Verification items for the finished model (mm, model axes). Coordinates: 2 decimals unless noted, no trailing zeros. Return JSON: item names as keys, results as strings. Group by question number.
Q1. Section check A-A, the plane y = 2. Count the separate pieces of the cut face and the enclosed holes in it, then the cut area to 3 significant figures.
Q2. Thickness scan on probe 1 along Z at (x, y) = (-91.5, 1.9) (3 decimals); probe 2 along X at (y, z) = (3.1, -29.5); probe 3 along Z at (x, y) = (-35.5, 0.8) (3 decimals). Record the ranges inside material, lowest first.
Q3. Mould release check, pull along Z, two halves, no side actions. Record for faces 1 (the face through (38.98, 2.46, 2.05)), 2 (the face through (153.225, 2.535, 1.55)): pulls with the +Z half, pulls with the -Z half, needs draft (parallel to the pull), parting line crosses it, or undercut.
Q4. Go/stop test with flat-tipped pins: pin 1 Ø1.5 at (y, z) = (3, -15.5) entering from -X; pin 2 Ø6 at (x, z) = (45.5, -21) entering from +Y; pin 3 Ø1.8 at (x, z) = (-105, -20.125) entering from +Y; pin 4 Ø2.5 at (x, y) = (-62.5, 3) entering from +Z (3 decimals). Record where each tip stops, or that it passes through.
from build123d import *

# Parameters (mm, degrees)
EXTRUDE_1_DEPTH      = 5
SKETCH_2_R           = 1.525
CUT_EXTRUDE_1_DEPTH  = 6
SKETCH_3_R           = 48.25
EXTRUDE_2_DEPTH      = 5
SKETCH_6_R           = 1.525
CUT_EXTRUDE_4_DEPTH  = 6
SKETCH_7_R           = 1.775
CUT_EXTRUDE_5_DEPTH  = 6
FILLET_1_R           = 40
SKETCH_9_R           = 14
CUT_EXTRUDE_7_DEPTH  = 6
SKETCH_10_R          = 8
CUT_EXTRUDE_8_DEPTH  = 6
SKETCH_11_R          = 15
CUT_EXTRUDE_9_DEPTH  = 6
SKETCH_12_R          = 3
CUT_EXTRUDE_10_DEPTH = 6
SKETCH_13_R          = 1.525
CUT_EXTRUDE_11_DEPTH = 6
SKETCH_18_R          = 1.525
CUT_EXTRUDE_13_DEPTH = 6
SKETCH_21_R          = 1.525
CUT_EXTRUDE_15_DEPTH = 6
CUT_EXTRUDE_16_DEPTH = 6


with BuildPart() as part:
    # 草图1 → 凸台-拉伸1 (new body)
    with BuildSketch(Plane(origin=(0, 0, 0), x_dir=(1, 0, 0), z_dir=(0, 1, 0))):
        with BuildLine():
            ThreePointArc((-78.875, 0), (-86.526835342, -18.473164658), (-105, -26.125))
            Line((-105, -26.125), (105, -26.125))
            Line((105, -26.125), (105, 26.125))
            Line((105, 26.125), (-105, 26.125))
            ThreePointArc((-105, 26.125), (-86.526835342, 18.473164658), (-78.875, 0))
        make_face()
        with BuildLine():
            ThreePointArc((-105, 26.125), (-131.125, 0), (-105, -26.125))
            Line((-105, -26.125), (-105, 26.125))
        make_face()
        with BuildLine():
            Line((-105, 26.125), (-105, -26.125))
            ThreePointArc((-105, -26.125), (-86.526835342, -18.473164658), (-78.875, 0))
            ThreePointArc((-78.875, 0), (-86.526835342, 18.473164658), (-105, 26.125))
        make_face()
    extrude(amount=EXTRUDE_1_DEPTH)

    # 草图2 → 切除-拉伸1 (cut, through all)
    with BuildSketch(Plane(origin=(0, 5, 0), x_dir=(1, 0, 0), z_dir=(0, 1, 0))):
        with Locations((-91.5, 0)):
            Circle(SKETCH_2_R)
        with Locations((-98.25, -11.691342951)):
            Circle(SKETCH_2_R)
        with Locations((-111.75, -11.691342951)):
            Circle(SKETCH_2_R)
        with Locations((-118.5, 0)):
            Circle(SKETCH_2_R)
        with Locations((-111.75, 11.691342951)):
            Circle(SKETCH_2_R)
        with Locations((-98.25, 11.691342951)):
            Circle(SKETCH_2_R)
    extrude(amount=-CUT_EXTRUDE_1_DEPTH, mode=Mode.SUBTRACT)

    # 草图3 → 凸台-拉伸2 (add)
    with BuildSketch(Plane(origin=(0, 5, 0), x_dir=(1, 0, 0), z_dir=(0, 1, 0))):
        with Locations((105, 0)):
            Circle(SKETCH_3_R)
    extrude(amount=-EXTRUDE_2_DEPTH)

    # 草图6 → 切除-拉伸4 (cut, through all)
    with BuildSketch(Plane(origin=(0, 5, 0), x_dir=(1, 0, 0), z_dir=(0, 1, 0))):
        with Locations((118.435028843, 13.435028843)):
            Circle(SKETCH_6_R)
        with Locations((124, 0)):
            Circle(SKETCH_6_R)
        with Locations((118.435028843, -13.435028843)):
            Circle(SKETCH_6_R)
        with Locations((105, -19)):
            Circle(SKETCH_6_R)
        with Locations((91.564971157, -13.435028843)):
            Circle(SKETCH_6_R)
        with Locations((86, 0)):
            Circle(SKETCH_6_R)
        with Locations((91.564971157, 13.435028843)):
            Circle(SKETCH_6_R)
        with Locations((105, 19)):
            Circle(SKETCH_6_R)
    extrude(amount=-CUT_EXTRUDE_4_DEPTH, mode=Mode.SUBTRACT)

    # 草图7 → 切除-拉伸5 (cut, through all)
    with BuildSketch(Plane(origin=(0, 5, 0), x_dir=(1, 0, 0), z_dir=(0, 1, 0))):
        with Locations((149.5, 0)):
            Circle(SKETCH_7_R)
        with Locations((136.466251763, -31.466251763)):
            Circle(SKETCH_7_R)
        with Locations((105, -44.5)):
            Circle(SKETCH_7_R)
        with Locations((73.533748237, -31.466251763)):
            Circle(SKETCH_7_R)
        with Locations((60.5, 0)):
            Circle(SKETCH_7_R)
        with Locations((73.533748237, 31.466251763)):
            Circle(SKETCH_7_R)
        with Locations((105, 44.5)):
            Circle(SKETCH_7_R)
        with Locations((136.466251763, 31.466251763)):
            Circle(SKETCH_7_R)
    extrude(amount=-CUT_EXTRUDE_5_DEPTH, mode=Mode.SUBTRACT)

    # 圆角1
    fillet_1_edges = [part.edges().sort_by_distance(p)[0] for p in [
        (64.43465919, 2.5, 26.125),
        (64.43465919, 2.5, -26.125),
    ]]
    fillet(fillet_1_edges, radius=FILLET_1_R)

    # 草图9 → 切除-拉伸7 (cut, through all)
    with BuildSketch(Plane(origin=(0, 5, 0), x_dir=(1, 0, 0), z_dir=(0, 1, 0))):
        with Locations((105, 0)):
            Circle(SKETCH_9_R)
    extrude(amount=-CUT_EXTRUDE_7_DEPTH, mode=Mode.SUBTRACT)

    # 草图10 → 切除-拉伸8 (cut, through all)
    with BuildSketch(Plane(origin=(0, 5, 0), x_dir=(1, 0, 0), z_dir=(0, 1, 0))):
        with Locations((-105, 0)):
            Circle(SKETCH_10_R)
    extrude(amount=-CUT_EXTRUDE_8_DEPTH, mode=Mode.SUBTRACT)

    # 草图11 → 切除-拉伸9 (cut, through all)
    with BuildSketch(Plane(origin=(0, 5, 0), x_dir=(1, 0, 0), z_dir=(0, 1, 0))):
        with Locations((105, 0)):
            Circle(SKETCH_11_R)
    extrude(amount=-CUT_EXTRUDE_9_DEPTH, mode=Mode.SUBTRACT)

    # 草图12 → 切除-拉伸10 (cut, through all)
    with BuildSketch(Plane(origin=(0, 5, 0), x_dir=(1, 0, 0), z_dir=(0, 1, 0))):
        with Locations((117.437211552, 30.026084807)):
            Circle(SKETCH_12_R)
        with Locations((135.026084807, 12.437211552)):
            Circle(SKETCH_12_R)
        with Locations((135.026084807, -12.437211552)):
            Circle(SKETCH_12_R)
        with Locations((117.437211552, -30.026084807)):
            Circle(SKETCH_12_R)
        with Locations((92.562788448, -30.026084807)):
            Circle(SKETCH_12_R)
        with Locations((74.973915193, -12.437211552)):
            Circle(SKETCH_12_R)
        with Locations((74.973915193, 12.437211552)):
            Circle(SKETCH_12_R)
        with Locations((92.562788448, 30.026084807)):
            Circle(SKETCH_12_R)
    extrude(amount=-CUT_EXTRUDE_10_DEPTH, mode=Mode.SUBTRACT)

    # 草图13 → 切除-拉伸11 (cut, through all)
    with BuildSketch(Plane(origin=(0, 5, 0), x_dir=(1, 0, 0), z_dir=(0, 1, 0))):
        with Locations((122.02941274, 41.112639197)):
            Circle(SKETCH_13_R)
        with Locations((146.112639197, 17.02941274)):
            Circle(SKETCH_13_R)
        with Locations((146.112639197, -17.02941274)):
            Circle(SKETCH_13_R)
        with Locations((122.02941274, -41.112639197)):
            Circle(SKETCH_13_R)
        with Locations((87.97058726, -41.112639197)):
            Circle(SKETCH_13_R)
        with Locations((63.887360803, -17.02941274)):
            Circle(SKETCH_13_R)
        with Locations((63.887360803, 17.02941274)):
            Circle(SKETCH_13_R)
        with Locations((87.97058726, 41.112639197)):
            Circle(SKETCH_13_R)
    extrude(amount=-CUT_EXTRUDE_11_DEPTH, mode=Mode.SUBTRACT)

    # 草图18 → 切除-拉伸13 (cut, through all)
    with BuildSketch(Plane(origin=(0, 5, 0), x_dir=(1, 0, 0), z_dir=(0, 1, 0))):
        with Locations((45, 20.125)):
            Circle(SKETCH_18_R)
        with Locations((25, 20.125)):
            Circle(SKETCH_18_R)
        with Locations((5, 20.125)):
            Circle(SKETCH_18_R)
        with Locations((-15, 20.125)):
            Circle(SKETCH_18_R)
        with Locations((-35, 20.125)):
            Circle(SKETCH_18_R)
        with Locations((-55, 20.125)):
            Circle(SKETCH_18_R)
        with Locations((-75, 20.125)):
            Circle(SKETCH_18_R)
    cut_extrude_13 = extrude(amount=-CUT_EXTRUDE_13_DEPTH, mode=Mode.SUBTRACT)

    # 镜向2: 切除-拉伸13 across plane
    add(cut_extrude_13.mirror(Plane.XY), mode=Mode.SUBTRACT)

    # 草图21 → 切除-拉伸15 (cut, through all)
    with BuildSketch(Plane(origin=(0, 5, 0), x_dir=(1, 0, 0), z_dir=(0, 1, 0))):
        with Locations((-105, 20.125)):
            Circle(SKETCH_21_R)
        with Locations((-87.571238749, 10.0625)):
            Circle(SKETCH_21_R)
        with Locations((-87.571238749, -10.0625)):
            Circle(SKETCH_21_R)
        with Locations((-105, -20.125)):
            Circle(SKETCH_21_R)
        with Locations((-122.428761251, -10.0625)):
            Circle(SKETCH_21_R)
        with Locations((-122.428761251, 10.0625)):
            Circle(SKETCH_21_R)
    extrude(amount=-CUT_EXTRUDE_15_DEPTH, mode=Mode.SUBTRACT)

    # 草图22 → 切除-拉伸16 (cut, through all)
    with BuildSketch(Plane.XZ):
        with BuildLine():
            Line((-69.181610021, -14), (-54, -14))
            ThreePointArc((-54, -14), (-52.585786438, -13.414213562), (-52, -12))
            Line((-52, -12), (-52, 5.003403224))
            ThreePointArc((-52, 5.003403224), (-53.287171355, 6.872059244), (-55.491875323, 6.335434762))
            Line((-55.491875323, 6.335434762), (-70.673485344, -10.667968461))
            ThreePointArc((-70.673485344, -10.667968461), (-71.006995333, -12.817293375), (-69.181610021, -14))
        make_face()
        with BuildLine():
            Line((-73.508124677, -6.335434762), (-58.326514656, 10.667968461))
            ThreePointArc((-58.326514656, 10.667968461), (-57.993004667, 12.817293375), (-59.818389979, 14))
            Line((-59.818389979, 14), (-75, 14))
            ThreePointArc((-75, 14), (-76.414213562, 13.414213562), (-77, 12))
            Line((-77, 12), (-77, -5.003403224))
            ThreePointArc((-77, -5.003403224), (-75.712828645, -6.872059244), (-73.508124677, -6.335434762))
        make_face()
        with BuildLine():
            Line((-42, 12), (-42, -5.003403224))
            ThreePointArc((-42, -5.003403224), (-40.712828645, -6.872059244), (-38.508124677, -6.335434762))
            Line((-38.508124677, -6.335434762), (-23.326514656, 10.667968461))
            ThreePointArc((-23.326514656, 10.667968461), (-22.993004667, 12.817293375), (-24.818389979, 14))
            Line((-24.818389979, 14), (-40, 14))
            ThreePointArc((-40, 14), (-41.414213562, 13.414213562), (-42, 12))
        make_face()
        with BuildLine():
            Line((-34.181610021, -14), (-19, -14))
            ThreePointArc((-19, -14), (-17.585786438, -13.414213562), (-17, -12))
            Line((-17, -12), (-17, 5.003403224))
            ThreePointArc((-17, 5.003403224), (-18.287171355, 6.872059244), (-20.491875323, 6.335434762))
            Line((-20.491875323, 6.335434762), (-35.673485344, -10.667968461))
            ThreePointArc((-35.673485344, -10.667968461), (-36.006995333, -12.817293375), (-34.181610021, -14))
        make_face()
        with BuildLine():
            Line((-7, 12), (-7, -5.003403224))
            ThreePointArc((-7, -5.003403224), (-5.712828645, -6.872059244), (-3.508124677, -6.335434762))
            Line((-3.508124677, -6.335434762), (11.673485344, 10.667968461))
            ThreePointArc((11.673485344, 10.667968461), (12.006995333, 12.817293375), (10.181610021, 14))
            Line((10.181610021, 14), (-5, 14))
            ThreePointArc((-5, 14), (-6.414213562, 13.414213562), (-7, 12))
        make_face()
        with BuildLine():
            Line((0.818389979, -14), (16, -14))
            ThreePointArc((16, -14), (17.414213562, -13.414213562), (18, -12))
            Line((18, -12), (18, 5.003403224))
            ThreePointArc((18, 5.003403224), (16.712828645, 6.872059244), (14.508124677, 6.335434762))
            Line((14.508124677, 6.335434762), (-0.673485344, -10.667968461))
            ThreePointArc((-0.673485344, -10.667968461), (-1.006995333, -12.817293375), (0.818389979, -14))
        make_face()
        with BuildLine():
            Line((28, 12), (28, -5.003403224))
            ThreePointArc((28, -5.003403224), (29.287171355, -6.872059244), (31.491875323, -6.335434762))
            Line((31.491875323, -6.335434762), (46.673485344, 10.667968461))
            ThreePointArc((46.673485344, 10.667968461), (47.006995333, 12.817293375), (45.181610021, 14))
            Line((45.181610021, 14), (30, 14))
            ThreePointArc((30, 14), (28.585786438, 13.414213562), (28, 12))
        make_face()
        with BuildLine():
            Line((35.818389979, -14), (51, -14))
            ThreePointArc((51, -14), (52.414213562, -13.414213562), (53, -12))
            Line((53, -12), (53, 5.003403224))
            ThreePointArc((53, 5.003403224), (51.712828645, 6.872059244), (49.508124677, 6.335434762))
            Line((49.508124677, 6.335434762), (34.326514656, -10.667968461))
            ThreePointArc((34.326514656, -10.667968461), (33.993004667, -12.817293375), (35.818389979, -14))
        make_face()
    extrude(amount=-CUT_EXTRUDE_16_DEPTH, mode=Mode.SUBTRACT)


solid = part.part
Numbers:
{
 "1": {"separate pieces": "1", "enclosed holes": "68", "area": "13,500 mm2"},
 "2": {"probe 1": "z = -26.125 to -1.525, 1.525 to 26.125", "probe 2": "x = 62.64 to 89.61, 95.52 to 114.48, 120.39 to 143.18", "probe 3": "z = -26.125 to -21.566, -18.684 to -13.504, -10.474 to -2.966, 14 to 18.684, 21.566 to 26.125"},
 "3": {"face 1": "undercut", "face 2": "parting line crosses it"},
 "4": {"pin 1": "stops at x = -126.56", "pin 2": "stops at y = 5", "pin 3": "passes through", "pin 4": "stops at z = 26.125"}
}
